Can you work these out from the model? Positions are in its coordinate system, mm. Give positions to 0.01 mm unless a question says otherwise; leave off trailing zeros. Order: outer loops, then holes, each group sorted by start corner. A loop starts at its lowest first (then second) coordinate and runs counter-clockwise, first axis right, second up. Notation, with made-up numbers: (18.5, 81.5) -> (71.5, 81.5) arc R30 ccw to (71.5, 120.5) -> close; hole circle Ø1 at (3.25, 59.5). An arc over 180 degrees is marked (long way). Answer as CSV lines item,"result".
```python
from build123d import *

# Parameters (mm, degrees)
SKETCH1_W           = 30
SKETCH1_H           = 55
BOSS_EXTRUDE1_DEPTH = 1.5
CHAMFER1_SIZE       = 3
CHAMFER2_SIZE       = 25


with BuildPart() as part:
    # Sketch1 → Boss-Extrude1 (new, symmetric)
    with BuildSketch(Plane.XY):
        Rectangle(SKETCH1_W, SKETCH1_H)
    extrude(amount=BOSS_EXTRUDE1_DEPTH, both=True)

    # Chamfer1
    chamfer1_edges = [part.edges().sort_by_distance(p)[0] for p in [
        (-15, 27.5, 0),
        (15, 27.5, 0),
    ]]
    chamfer(chamfer1_edges, length=CHAMFER1_SIZE)

    # Chamfer2
    chamfer2_edges = [part.edges().sort_by_distance(p)[0] for p in [
        (15, -27.5, 0),
    ]]
    chamfer(chamfer2_edges, length=CHAMFER2_SIZE)


solid = part.part
```
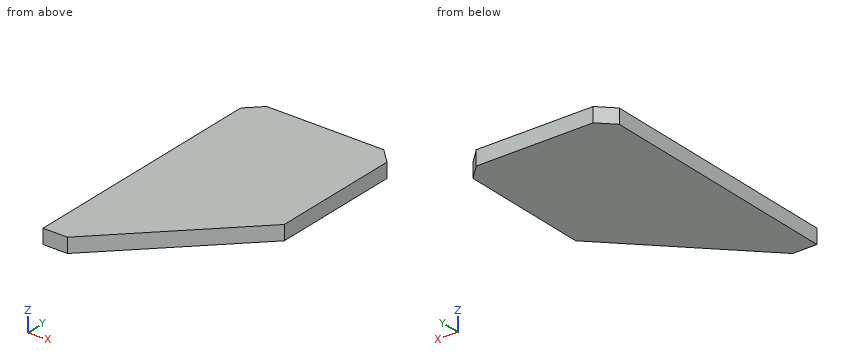
Item 1: For pin 1 (1 mm diameter, centred on y = -10.5, z = 1, fed in from +X), with a flat end and sliding along its axis, tell me the tip position at first contact or that it passes through.
Numbers:
pin 1,"stops at x = 7.5"
Item 2: Imagine slicing it at B-B, the plane x = 10. Please give me the cut outline in (y, z), then the cut area to 3 significant figures.
Numbers:
outline,"(-7.5, -1.5) -> (27.5, -1.5) -> (27.5, 1.5) -> (-7.5, 1.5) -> close"
area,"105 mm²"
Item 3: Imagine slicing it at A-A, the plane z = -0.05. Please give me the cut outline in (x, y), then the cut area to 3 significant figures.
Numbers:
outline,"(-15, -27.5) -> (-10, -27.5) -> (15, -2.5) -> (15, 24.5) -> (12, 27.5) -> (-12, 27.5) -> (-15, 24.5) -> close"
area,"1,330 mm²"
Item 4: Please list where these lines run through material, in increasing order: line 1 along Y through (x, z) = (5.5, 1.15); line 2 along X through (y, z) = (-18, -0.95); line 3 along Y through (x, z) = (2, -0.7).
Numbers:
line 1,"y = -12 to 27.5"
line 2,"x = -15 to -0.5"
line 3,"y = -15.5 to 27.5"
Item 5: Imagine slicing it at C-C, the plane y = -20.5. Please give me the cut outline in (x, z), then the cut area to 3 significant figures.
Numbers:
outline,"(-15, -1.5) -> (-3, -1.5) -> (-3, 1.5) -> (-15, 1.5) -> close"
area,"36.0 mm²"
